Design review of the part built by this model. Coordinates are the model's own, in mm. A direction names the side the tool comes from. Give positions to 0.01 mm unless a question says otherwise; leave off trailing zeros. Loops run counter-clockwise (first coordinate to the right, second up) from the corner with the lowest first, then second, coordinate; pieces in that order, holes last. Notation, with made-up numbers: (22.25, 36.5) - (55.25, 36.5) arc R30 cw to (55.25, 72.5) - close; hole circle Ø2 at (48, 27). An arc over 180 degrees is marked (long way). Write each question's results on one line, items separated by ' | '.
from build123d import *

# Parameters (mm, degrees)
CUT_EXTRUDE2_REACH              = 24
M5X0_8_TAPPED_HOLE1_D           = 4.2
M5X0_8_TAPPED_HOLE1_DEPTH       = 7
M5X0_8_TAPPED_HOLE1_CSINK_D     = 5.5
M5X0_8_TAPPED_HOLE1_CSINK_ANGLE = 90


with BuildPart() as part:
    # Sketch1 → Revolve1 (revolve)
    with BuildSketch(Plane(origin=(0, 0, 0), x_dir=(0, 0, -1), z_dir=(1, 0, 0))):
        Polygon((-12.5, 3.1), (-13.5, 4.1), (-13.5, 5), (-12.5, 6), (-1.5, 6), (-1.5, 9), (8.5, 9), (8.5, 5.75), (9.85, 5.75), (9.85, 5.05), (13.5, 5.05), (13.5, 2.25), (-8, 2.25), (-8, 4.15), (-11.5, 4.15), (-11.5, 3.1), align=None)
    revolve(axis=Axis((0, 0, 0), (0, 0, -1)))

    # Sketch2 → Cut-Extrude2 (cut, up to next)
    with BuildSketch(Plane(origin=(0, 0, -8.5), x_dir=(-1, 0, 0), z_dir=(0, 0, -1)), mode=Mode.PRIVATE) as cut_extrude2_sk1:
        with BuildLine():
            ThreePointArc((4.242180306, 7.9375), (0, 9), (-4.242180306, 7.9375))
            Line((-4.242180306, 7.9375), (4.242180306, 7.9375))
        make_face()
    cut_extrude2_tool1 = extrude(cut_extrude2_sk1.sketch, amount=-CUT_EXTRUDE2_REACH, mode=Mode.PRIVATE) & part.part
    add(cut_extrude2_tool1.solids().sort_by_distance((0, 8.364726, -8.5))[0], mode=Mode.SUBTRACT)
    # Sketch2 → Cut-Extrude2 (cut, up to next)
    with BuildSketch(Plane(origin=(0, 0, -8.5), x_dir=(-1, 0, 0), z_dir=(0, 0, -1)), mode=Mode.PRIVATE) as cut_extrude2_sk2:
        with BuildLine():
            Line((-7.9375, -4.242180306), (-7.9375, 4.242180306))
            ThreePointArc((-7.9375, 4.242180306), (-9, 0), (-7.9375, -4.242180306))
        make_face()
    cut_extrude2_tool2 = extrude(cut_extrude2_sk2.sketch, amount=-CUT_EXTRUDE2_REACH, mode=Mode.PRIVATE) & part.part
    add(cut_extrude2_tool2.solids().sort_by_distance((8.364726, 0, -8.5))[0], mode=Mode.SUBTRACT)
    # Sketch2 → Cut-Extrude2 (cut, up to next)
    with BuildSketch(Plane(origin=(0, 0, -8.5), x_dir=(-1, 0, 0), z_dir=(0, 0, -1)), mode=Mode.PRIVATE) as cut_extrude2_sk3:
        with BuildLine():
            Line((4.242180306, -7.9375), (-4.242180306, -7.9375))
            ThreePointArc((-4.242180306, -7.9375), (0, -9), (4.242180306, -7.9375))
        make_face()
    cut_extrude2_tool3 = extrude(cut_extrude2_sk3.sketch, amount=-CUT_EXTRUDE2_REACH, mode=Mode.PRIVATE) & part.part
    add(cut_extrude2_tool3.solids().sort_by_distance((0, -8.364726, -8.5))[0], mode=Mode.SUBTRACT)
    # Sketch2 → Cut-Extrude2 (cut, up to next)
    with BuildSketch(Plane(origin=(0, 0, -8.5), x_dir=(-1, 0, 0), z_dir=(0, 0, -1)), mode=Mode.PRIVATE) as cut_extrude2_sk4:
        with BuildLine():
            ThreePointArc((9, 0), (8.730335045, 2.186606961), (7.9375, 4.242180306))
            Line((7.9375, 4.242180306), (7.9375, -4.242180306))
            ThreePointArc((7.9375, -4.242180306), (8.730335045, -2.186606961), (9, 0))
        make_face()
    cut_extrude2_tool4 = extrude(cut_extrude2_sk4.sketch, amount=-CUT_EXTRUDE2_REACH, mode=Mode.PRIVATE) & part.part
    add(cut_extrude2_tool4.solids().sort_by_distance((-8.364726, 0, -8.5))[0], mode=Mode.SUBTRACT)

    # M5x0.8 Tapped Hole1
    with Locations(Plane(origin=(0, 7.9375, 0), x_dir=(1, 0, 0), z_dir=(0, 1, 0))):
        with Locations((0, 4.5)):
            CounterSinkHole(M5X0_8_TAPPED_HOLE1_D / 2, M5X0_8_TAPPED_HOLE1_CSINK_D / 2, depth=M5X0_8_TAPPED_HOLE1_DEPTH, counter_sink_angle=M5X0_8_TAPPED_HOLE1_CSINK_ANGLE)


solid = part.part
(1) Insertion check: P1, Ø3, axis at x = 6, z = 10.5, coming from the -Y side; P2, Ø4, axis at x = -0.5, y = -1.5, coming from the -Z side; P3, Ø1.5, axis at y = -3.5, z = 7, coming from the -X side; P4, Ø5.5, axis at x = 0, y = 0, coming from the +Z side. Each pin has a flat end and moves straight along its axis. Give the tip position at first contact, or say it passes through.
Answers below:
P1: y = -3.97 | P2: z = -13.5 | P3: x = -5.33 | P4: z = 8
(2) Tool access review of faces 4 (the cylindrical face through (0, -6, 7)), 5 (the flat face through (-3, -2, 11.5)), 6 (the cylindrical face through (5.7, -0.75, -9.18)), 7 (the flat face through (-1.1, 2.2, -13.5)), 8 (the flat face through (0, -7.938, -4)): name each direction out of +Z, -Z, +X, -X, +Y, -Y from which nothing blocks a thin tool from reaching the whole face with its end or side.
Answers below:
face 4: +Z | face 5: none | face 6: -Z | face 7: -Z, +X, -X, +Y, -Y | face 8: +Z, -Z, +X, -X, -Y
(3) Take a section at C-C on x = 0. Count the separate pieces of the cut face and the enclosed holes in it, plus the area to 3 significant figures.
Answers below:
separate pieces: 3 | enclosed holes: 0 | area: 191 mm2
(4) Draft analysis for pull direction Z (two halves, no side actions). For faces 1 (the flat face through (-7.938, 0, -4)), 2 (the flat face through (4, -5, -8.5)), 3 (the cylindrical face through (-1.13, 4.07, -6.27)), state which applies: pulls with the +Z half, pulls with the -Z half, needs draft (parallel to the pull), parting line crosses it, or undercut.
Answers below:
face 1: needs draft | face 2: pulls with the -Z half | face 3: undercut
(5) Take a section at B-B on z = -1. Give the boundary of the cut face in (x, y), plus the area to 3 significant figures.
Answers below:
outline: (-7.94, -4.24) arc R9 ccw to (-4.24, -7.94) - (4.24, -7.94) arc R9 ccw to (7.94, -4.24) - (7.94, 4.24) arc R9 ccw to (4.24, 7.94) - (-4.24, 7.94) arc R9 ccw to (-7.94, 4.24) - close; hole circle Ø4.5 at (0, 0) | area: 214 mm2
(6) Wall thickness on line 1 along X through (y, z) = (0, 11.85); line 2 along Z through (x, y) = (0, 2.75); line 3 along Z through (x, y) = (0, 5): over which ranges is each line inside the solid? List them lowest first. Write a range as from..to.
Answers below:
line 1: -6..-3.1, 3.1..6 | line 2: -13.5..-6.6, -2.4..8 | line 3: -13.5..-6.6, -2.4..13.5
(7) Take a section at D-D on z = -4.5. Give the boundary of the cut face in (x, y), plus the area to 3 significant figures.
Answers below:
outline: (-7.94, -4.24) arc R9 ccw to (-4.24, -7.94) - (4.24, -7.94) arc R9 ccw to (7.94, -4.24) - (7.94, 4.24) arc R9 ccw to (4.24, 7.94) - (2.75, 7.94) - (2.1, 7.29) - (2.1, 0.94) - (2.05, 0.94) arc R2.25 cw (long way) to (-2.05, 0.94) - (-2.1, 0.94) - (-2.1, 7.29) - (-2.75, 7.94) - (-4.24, 7.94) arc R9 ccw to (-7.94, 4.24) - close | area: 188 mm2
